Could you check a few things on this model? Use its own coordinates, in mm. Round coordinates to 2 decimals unless told otherwise and drop trailing zeros. Loops run counter-clockwise (first coordinate to the right, second up) from the corner with the lowest first, then second, coordinate; pieces in that order, holes last.
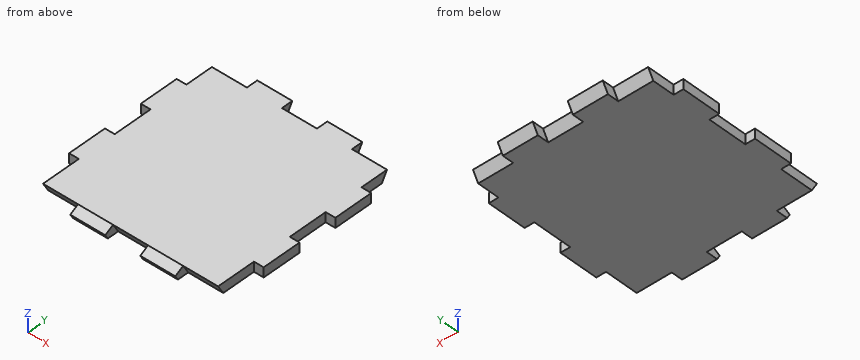
from build123d import *

# Parameters (mm, degrees)
ESQUISSE1_W             = 90
ESQUISSE1_H             = 100
BOSS_EXTRU_1_DEPTH      = 5
ENL_V_MAT_EXTRU_1_DEPTH = 135.629120178
BOSS_EXTRU_2_DEPTH      = 90
ESQUISSE10_W            = 18
ESQUISSE10_H            = 15
BOSS_EXTRU_4_DEPTH      = 5
ENL_V_MAT_EXTRU_3_DEPTH = 126.676901627
ESQUISSE12_W            = 18
ESQUISSE12_H            = 12
BOSS_EXTRU_5_DEPTH      = 5
ENL_V_MAT_EXTRU_4_DEPTH = 134.240384268
ESQUISSE14_W            = 5
ESQUISSE14_H            = 20
BOSS_EXTRU_6_DEPTH      = 5


with BuildPart() as part:
    # Esquisse1 → Boss.-Extru.1 (new body)
    with BuildSketch(Plane.XY):
        with Locations((-45, -50)):
            Rectangle(ESQUISSE1_W, ESQUISSE1_H)
    extrude(amount=BOSS_EXTRU_1_DEPTH)

    # Esquisse2 → Enlèv. mat.-Extru.1 (cut, through all)
    with BuildSketch(Plane(origin=(0, 0, 0), x_dir=(0, 0, -1), z_dir=(1, 0, 0))):
        Polygon((0, -11.547005384), (-5, -8.660254038), (-5, 0), (0, 0), align=None)
    extrude(amount=-ENL_V_MAT_EXTRU_1_DEPTH, mode=Mode.SUBTRACT)

    # Esquisse3 → Boss.-Extru.2 (add, through all)
    with BuildSketch(Plane(origin=(0, 0, 0), x_dir=(0, 0, -1), z_dir=(1, 0, 0))):
        Polygon((-5, -100), (-5, -102.886751346), (0, -100), align=None)
    extrude(amount=-BOSS_EXTRU_2_DEPTH)

    # Esquisse10 → Boss.-Extru.4 (add, through all)
    with BuildSketch(Plane(origin=(0, 0, 0), x_dir=(-1, 0, 0), z_dir=(0, 0, -1))):
        with Locations((27, -4.047005384)):
            Rectangle(ESQUISSE10_W, ESQUISSE10_H)
        with Locations((63, -4.047005384)):
            Rectangle(ESQUISSE10_W, ESQUISSE10_H)
    extrude(amount=-BOSS_EXTRU_4_DEPTH)

    # Esquisse11 → Enlèv. mat.-Extru.3 (cut, through all)
    with BuildSketch(Plane(origin=(-18, 0, 0), x_dir=(0, 0, -1), z_dir=(1, 0, 0))):
        Polygon((0, -5.773502692), (-5, -2.886751346), (-5, 3.452994616), (0, 3.452994616), align=None)
    extrude(amount=-ENL_V_MAT_EXTRU_3_DEPTH, mode=Mode.SUBTRACT)

    # Esquisse12 → Boss.-Extru.5 (add)
    with BuildSketch(Plane(origin=(0, 0, 0), x_dir=(-1, 0, 0), z_dir=(0, 0, -1))):
        with Locations((27, -106)):
            Rectangle(ESQUISSE12_W, ESQUISSE12_H)
        with Locations((63, -106)):
            Rectangle(ESQUISSE12_W, ESQUISSE12_H)
    extrude(amount=-BOSS_EXTRU_5_DEPTH)

    # Esquisse13 → Enlèv. mat.-Extru.4 (cut, through all)
    with BuildSketch(Plane(origin=(-18, 0, 0), x_dir=(0, 0, -1), z_dir=(1, 0, 0))):
        Polygon((-2.5, -107.216878365), (-5, -102.886751346), (-5, -112), (0, -112), (0, -105.773502692), align=None)
    extrude(amount=-ENL_V_MAT_EXTRU_4_DEPTH, mode=Mode.SUBTRACT)

    # Esquisse14 → Boss.-Extru.6 (add, through all)
    with BuildSketch(Plane.XY.offset(5)):
        with Locations((2.5, -32.886751346)):
            Rectangle(ESQUISSE14_W, ESQUISSE14_H)
        with Locations((2.5, -72.886751346)):
            Rectangle(ESQUISSE14_W, ESQUISSE14_H)
        with Locations((-92.5, -72.886751346)):
            Rectangle(ESQUISSE14_W, ESQUISSE14_H)
        with Locations((-92.5, -32.886751346)):
            Rectangle(ESQUISSE14_W, ESQUISSE14_H)
    extrude(amount=-BOSS_EXTRU_6_DEPTH)


solid = part.part
Item 1: If we section it at C-C, the plane x = -38: Please give me the cut outline in (y, z).
Results list:
outline: (-102.89, 5) - (-100, 0) - (-11.55, 0) - (-8.66, 5) - close
Item 2: If I drill on line 1 along X through (y, z) = (-51, 2.4); line 2 along Y through (x, z) = (-82, 3.55); line 3 along Y through (x, z) = (-9.5, 2.95), over which ranges is the centre line in solid material (lowest first)?
Results list:
line 1: x = -90 to 0
line 2: y = -102.05 to -9.5
line 3: y = -101.7 to -9.84
Item 3: Will these pins go through, and if not, where does the flat tip stop? pin 1 (1 mm diameter, centred on x = -13.5, z = 2, fed in from -Y); pin 2 (1.5 mm diameter, centred on y = -103, z = 2, fed in from -X); pin 3 (2.5 mm diameter, centred on x = -92.5, z = 2.5, fed in from -Y).
Results list:
pin 1: stops at y = -101.44
pin 2: stops at x = -72
pin 3: stops at y = -82.89
Item 4: If we section it at A-A, the plane y = -88: Please give me the cut outline in (x, z).
Results list:
outline: (-90, 0) - (0, 0) - (0, 5) - (-90, 5) - close
Item 5: If we section it at B-B, the plane x = -24: Please give me the cut outline in (y, z), then the cut area to 3 significant figures.
Results list:
outline: (-107.22, 2.5) - (-105.77, 0) - (-5.77, 0) - (-2.89, 5) - (-102.89, 5) - close
area: 507 mm2
